```python
from build123d import *

# Parameters (mm, degrees)
EXTRUDE_1_DEPTH             = 1
SKETCH_2_W                  = 6
SKETCH_2_H                  = 6
EXTRUDE_2_DEPTH             = 1
SKETCH_3_W                  = 20
SKETCH_3_H                  = 1
EXTRUDE_3_DEPTH             = 1.5
FILLET_1_R                  = 2
HOLE_WIZARD_M2_1_AT_2_COUNT = 2
HOLE_WIZARD_M2_1_AT_2_PITCH = 15.532224567
HOLE_WIZARD_M2_1_AT_3_COUNT = 2
HOLE_WIZARD_M2_1_AT_3_PITCH = 27.735356497
HOLE_WIZARD_M2_1_AT_4_COUNT = 2
HOLE_WIZARD_M2_1_AT_4_PITCH = 33
CUT_EXTRUDE_1_DEPTH         = 37.932370625


with BuildPart() as part:
    # 草图1 → 凸台-拉伸1 (new body)
    with BuildSketch(Plane.XY):
        Polygon((-8, 5), (-15, 5), (-16.499999995, 5), (-18, 5), (-18, -5), (-9.5, -5), (-8.000000003, -5), (-6.5, -5), (6.5, -5), (8, -5), (9.5, -5), (18, -5), (18, 5), (16.500000001, 5), (15, 5), (8, 5), (8, 1), (-8, 1), align=None)
        with BuildLine():
            ThreePointArc((-6.5, -6.5), (-6.939339829, -5.439339827), (-8.000000003, -5))
            ThreePointArc((-8.000000003, -5), (-9.060660173, -5.439339829), (-9.5, -6.5))
            Line((-9.5, -6.5), (-6.5, -6.5))
        make_face()
        with BuildLine():
            Line((-6.5, -6.5), (-9.5, -6.5))
            ThreePointArc((-9.5, -6.5), (-8, -8), (-6.5, -6.5))
        make_face()
        with BuildLine():
            Line((-8.000000003, -5), (-9.5, -5))
            Line((-9.5, -5), (-9.5, -6.5))
            ThreePointArc((-9.5, -6.5), (-9.060660173, -5.439339829), (-8.000000003, -5))
        make_face()
        with BuildLine():
            Line((-6.5, -5), (-8.000000003, -5))
            ThreePointArc((-8.000000003, -5), (-6.939339829, -5.439339827), (-6.5, -6.5))
            Line((-6.5, -6.5), (-6.5, -5))
        make_face()
        with BuildLine():
            ThreePointArc((9.5, -6.5), (9.060660172, -5.439339828), (8, -5))
            ThreePointArc((8, -5), (6.939339828, -5.439339828), (6.5, -6.5))
            Line((6.5, -6.5), (9.5, -6.5))
        make_face()
        with BuildLine():
            ThreePointArc((6.5, -6.5), (8, -8), (9.5, -6.5))
            Line((9.5, -6.5), (6.5, -6.5))
        make_face()
        with BuildLine():
            Line((8, -5), (6.5, -5))
            Line((6.5, -5), (6.5, -6.5))
            ThreePointArc((6.5, -6.5), (6.939339828, -5.439339828), (8, -5))
        make_face()
        with BuildLine():
            Line((9.5, -6.5), (9.5, -5))
            Line((9.5, -5), (8, -5))
            ThreePointArc((8, -5), (9.060660172, -5.439339828), (9.5, -6.5))
        make_face()
        with BuildLine():
            Line((-18, 5), (-16.499999995, 5))
            ThreePointArc((-16.499999995, 5), (-17.56066017, 5.439339826), (-18, 6.5))
            Line((-18, 6.5), (-18, 5))
        make_face()
        with BuildLine():
            ThreePointArc((-18, 6.5), (-17.56066017, 5.439339826), (-16.499999995, 5))
            ThreePointArc((-16.499999995, 5), (-15.439339826, 5.43933983), (-15, 6.5))
            Line((-15, 6.5), (-18, 6.5))
        make_face()
        with BuildLine():
            Line((-18, 6.5), (-15, 6.5))
            ThreePointArc((-15, 6.5), (-16.5, 8), (-18, 6.5))
        make_face()
        with BuildLine():
            Line((-16.499999995, 5), (-15, 5))
            Line((-15, 5), (-15, 6.5))
            ThreePointArc((-15, 6.5), (-15.439339826, 5.43933983), (-16.499999995, 5))
        make_face()
        with BuildLine():
            Line((15, 6.5), (15, 5))
            Line((15, 5), (16.500000001, 5))
            ThreePointArc((16.500000001, 5), (15.439339829, 5.439339828), (15, 6.5))
        make_face()
        with BuildLine():
            ThreePointArc((15, 6.5), (15.439339829, 5.439339828), (16.500000001, 5))
            ThreePointArc((16.500000001, 5), (17.560660172, 5.439339829), (18, 6.5))
            Line((18, 6.5), (15, 6.5))
        make_face()
        with BuildLine():
            ThreePointArc((18, 6.5), (16.5, 8), (15, 6.5))
            Line((15, 6.5), (18, 6.5))
        make_face()
        with BuildLine():
            ThreePointArc((18, 6.5), (17.560660172, 5.439339829), (16.500000001, 5))
            Line((16.500000001, 5), (18, 5))
            Line((18, 5), (18, 6.5))
        make_face()
    extrude(amount=EXTRUDE_1_DEPTH)

    # 草图2 → 凸台-拉伸2 (add)
    with BuildSketch(Plane.XY.offset(1)):
        with Locations((-13, 0)):
            Rectangle(SKETCH_2_W, SKETCH_2_H)
        with Locations((13, 0)):
            Rectangle(SKETCH_2_W, SKETCH_2_H)
    extrude(amount=EXTRUDE_2_DEPTH)

    # 草图3 → 凸台-拉伸3 (add)
    with BuildSketch(Plane(origin=(0, 0, 0), x_dir=(-1, 0, 0), z_dir=(0, 0, -1))):
        with Locations((2, 0.5)):
            Rectangle(SKETCH_3_W, SKETCH_3_H)
    extrude(amount=EXTRUDE_3_DEPTH)

    # 圆角1
    fillet_1_edges = [part.edges().sort_by_distance(p)[0] for p in [
        (18, -5, 0.5),
        (-18, -5, 0.5),
    ]]
    fillet(fillet_1_edges, radius=FILLET_1_R)

    # 草图5 → M2 螺纹孔1 (revolve, cut)
    with BuildSketch(Plane(origin=(-16.5, 6.5, 1), x_dir=(0, -1, 0), z_dir=(1, 0, 0))):
        Polygon((0, 0), (0, 1), (0.8, 1), (0.8, 0.225), (1.025, 0), align=None)
    hole_wizard_m2_1 = revolve(axis=Axis((-16.5, 6.5, 7.35), (0, 0, -1)), mode=Mode.SUBTRACT)

    # M2 螺纹孔1 at 2: M2 螺纹孔1 ×2
    with Locations(*[Vector(0.5472493629827028, -0.8369696139735456, 0) * (i * HOLE_WIZARD_M2_1_AT_2_PITCH) for i in range(1, HOLE_WIZARD_M2_1_AT_2_COUNT)]):
        add(hole_wizard_m2_1, mode=Mode.SUBTRACT)

    # M2 螺纹孔1 at 3: M2 螺纹孔1 ×2
    with Locations(*[Vector(0.8833490206949295, -0.46871580689935033, 0) * (i * HOLE_WIZARD_M2_1_AT_3_PITCH) for i in range(1, HOLE_WIZARD_M2_1_AT_3_COUNT)]):
        add(hole_wizard_m2_1, mode=Mode.SUBTRACT)

    # M2 螺纹孔1 at 4: M2 螺纹孔1 ×2
    with Locations(*[(i * HOLE_WIZARD_M2_1_AT_4_PITCH, 0, 0) for i in range(1, HOLE_WIZARD_M2_1_AT_4_COUNT)]):
        add(hole_wizard_m2_1, mode=Mode.SUBTRACT)

    # 草图7 → 切除-拉伸1 (cut, through all)
    with BuildSketch(Plane.ZY.offset(18)):
        Polygon((0, 52.66451622), (0, 8.533671193), (0, -8.947821263), (0, -53.078666291), (-88.261690055, -53.078666291), (-88.261690055, 52.66451622), align=None)
    extrude(amount=-CUT_EXTRUDE_1_DEPTH, mode=Mode.SUBTRACT)


solid = part.part
```
Geometry: final body of the model. Coordinates: model frame, mm. A direction names the side the tool comes from. Give positions to 0.01 mm unless a question says otherwise; leave off trailing zeros. Loops run counter-clockwise (first coordinate to the right, second up) from the corner with the lowest first, then second, coordinate; pieces in that order, holes last. Notation, with made-up numbers: (63.25, 83.25) - (79.25, 83.25) arc R6 ccw to (79.25, 92.25) - close; hole circle Ø7 at (71, 59). An arc over 180 degrees is marked (long way). Answer as CSV lines item,"result". Start each with the question number.
(1) Section query A-A (z = 1.4). Output: boundary loops of the cut face in (x, y), and give its area (3 significant figures).
(2) Reachability of faces 1 (the face through (8, 3, 0.5)), 2 (the face through (-10, 0, 1.5)), 3 (the face through (-12.8, -5, 0.5)), 4 (the face through (6.5, -5.7, 0.5)), 5 (the face through (13, -3, 1.5)) from +Z, -Z, +X, -X, +Y, -Y: full face, straight path, thin tool, end or side. Return the list, or none.
(3) Section query C-C (y = -1.5). Output: boundary loops of the cut face in (x, z).
(4) Pin query (flat end, axial travel): P1, Ø0.5, axis at x = -14, z = 0.5, coming from the -Y side; P2, Ø1.1, axis at x = 12, z = 0.5, coming from the +Y side; P3, Ø0.5, axis at y = 0.5, z = 1.5, coming from the +X side. Return the tip coordinate at first contact, or that it passes through.
(5) Section query B-B (x = -10.5). Output: boundary loops of the cut face in (y, z), and give its area (3 significant figures).
(6) Mould query, pull axis Y, two halves, no side actions, for faces 6 (the face through (8.78, -6.33, 0.39)), 7 (the face through (0, 0, 1)), 8 (the face through (-17.4, -4.43, 0.51)), 9 (the face through (-8.793, -6.396, 0.393)). Classes: +Y half, -Y half, draft (parallel to the pull), parting line (faces both ways), or undercut.
(7) Ray query, line 1 along X through (y, z) = (-6.5, 0.3); line 2 along X through (y, z) = (6.5, 0.6); line 3 along X through (y, z) = (3, 0.65). Return the intervals inside material, ascending. Write a range as [from, to].
Worked answers:
1,outline,"(-16, -3) - (-10, -3) - (-10, 3) - (-16, 3) - close; (10, -3) - (16, -3) - (16, 3) - (10, 3) - close"
1,area,"72.0 mm^2"
2,face 1,"+Z, -Z, +Y"
2,face 2,"+Z, +Y, -Y"
2,face 3,"+Z, -Z, -X, -Y"
2,face 4,"+Z, -Z, -Y"
2,face 5,"+Z, +X, -X, -Y"
3,outline,"(-18, 0) - (18, 0) - (18, 1) - (16, 1) - (16, 2) - (10, 2) - (10, 1) - (-10, 1) - (-10, 2) - (-16, 2) - (-16, 1) - (-18, 1) - close"
4,P1,"stops at y = -5"
4,P2,"stops at y = 5"
4,P3,"stops at x = 16"
5,outline,"(-5, 0) - (5, 0) - (5, 1) - (3, 1) - (3, 2) - (-3, 2) - (-3, 1) - (-5, 1) - close"
5,area,"16.0 mm^2"
6,face 6,"undercut"
6,face 7,"draft"
6,face 8,"-Y half"
6,face 9,"undercut"
7,line 1,"x = [-9.5, -8.8], [-7.2, -6.5], [6.5, 7.2], [8.8, 9.5]"
7,line 2,"x = [-18, -17.3], [-15.7, -15], [15, 15.7], [17.3, 18]"
7,line 3,"x = [-18, -8], [8, 18]"
